Design review of the part built by this model. Coordinates are the model's own, in mm. Give positions to 0.01 mm unless a question says otherwise; leave off trailing zeros. Write each loop counter-clockwise with the first axis right and the second up, starting at its lowest first coordinate (ties: lowest second). Pieces come first, ordered by that corner, then holes. Notation, with made-up numbers: (80, -33.5) - (85, -33.5) arc R14 ccw to (85, -17.5) - close; hole circle Ø4 at (-29, -34). An arc over 180 degrees is marked (long way). Write each question's results on one line, items separated by ' | '. Start each with the question number.
from build123d import *

# Parameters (mm, degrees)
SKETCH1_W           = 3
SKETCH1_H           = 40
EXTRUDE_THIN1_DEPTH = 90
CAVITY1_START       = -65.602294015
CAVITY1_OUTLINE_W   = 3
CAVITY1_OUTLINE_H   = 3
CAVITY1_DEPTH       = 10
CAVITY1_START_2     = -35.602294015
CAVITY1_2_OUTLINE_W = 3
CAVITY1_2_OUTLINE_H = 3
CAVITY1_2_DEPTH     = 10
FILLET1_R           = 2


# Read off the part's stored shape, not the designer's step: Cavity1
with BuildPart() as part:
    # Sketch1 → Extrude-Thin1 (new body)
    with BuildSketch(Plane.XY.offset(1.5)):
        with Locations((84.585106383, -45.602294015)):
            Rectangle(SKETCH1_W, SKETCH1_H)
    extrude(amount=-EXTRUDE_THIN1_DEPTH)

    # Cavity1 outline → Cavity1 (cut)
    with BuildSketch(Plane(origin=(0, 0, 0), x_dir=(1, 0, 0), z_dir=(0, 1, 0)).offset(CAVITY1_START)):
        with Locations((84.585106383, 87)):
            Rectangle(CAVITY1_OUTLINE_W, CAVITY1_OUTLINE_H)
        with Locations((84.585106383, 0)):
            Rectangle(CAVITY1_OUTLINE_W, CAVITY1_OUTLINE_H)
    extrude(amount=CAVITY1_DEPTH, mode=Mode.SUBTRACT)

    # Cavity1 2 outline → Cavity1 2 (cut)
    with BuildSketch(Plane(origin=(0, 0, 0), x_dir=(1, 0, 0), z_dir=(0, 1, 0)).offset(CAVITY1_START_2)):
        with Locations((84.585106383, 87)):
            Rectangle(CAVITY1_2_OUTLINE_W, CAVITY1_2_OUTLINE_H)
        with Locations((84.585106383, 0)):
            Rectangle(CAVITY1_2_OUTLINE_W, CAVITY1_2_OUTLINE_H)
    extrude(amount=CAVITY1_2_DEPTH, mode=Mode.SUBTRACT)

    # Fillet1
    fillet1_edges = [part.edges().sort_by_distance(p)[0] for p in [
        (84.585106383, -65.602294015, -85.5),
        (84.585106383, -25.602294015, -85.5),
        (84.585106383, -65.602294015, -1.5),
        (84.585106383, -25.602294015, -1.5),
    ]]
    fillet(fillet1_edges, radius=FILLET1_R)


solid = part.part
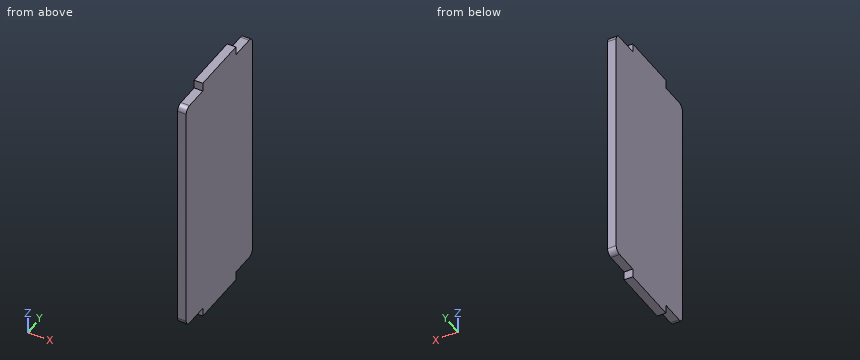
Q1. Insertion check: P1, Ø0.9, axis at x = 84.5, y = -30, coming from the +Z side; P2, Ø0.9, axis at x = 84.5, y = -30.5, coming from the -Z side; P3, Ø0.9, axis at x = 84.5, z = -87, coming from the +Y side. Each pin has a flat end and moves straight along its axis. Give the tip position at first contact, or say it passes through.
Q2. Add section A-A on x = 84.8. State the section outline as (y, z) points, plus the area to 3 significant figures.
Q3. For line 1 along Z through (x, y) = (84.7, -61); line 2 along Y through (x, z) = (84.9, -2.5), list the stretches that pass through material, from the lowest coordinate up. Write a range as [from, to].
Q4. Add section B-B on y = -61. State the section outline as (x, z) points.
Result:
1) P1: stops at z = -1.5 | P2: stops at z = -85.5 | P3: stops at y = -35.6
2) outline: (-65.6, -83.5) arc R2 ccw to (-63.6, -85.5) - (-55.6, -85.5) - (-55.6, -88.5) - (-35.6, -88.5) - (-35.6, -85.5) - (-27.6, -85.5) arc R2 ccw to (-25.6, -83.5) - (-25.6, -3.5) arc R2 ccw to (-27.6, -1.5) - (-35.6, -1.5) - (-35.6, 1.5) - (-55.6, 1.5) - (-55.6, -1.5) - (-63.6, -1.5) arc R2 ccw to (-65.6, -3.5) - close | area: 3,480 mm²
3) line 1: z = [-85.5, -1.5] | line 2: y = [-65.33, -25.87]
4) outline: (83.09, -85.5) - (86.09, -85.5) - (86.09, -1.5) - (83.09, -1.5) - close
